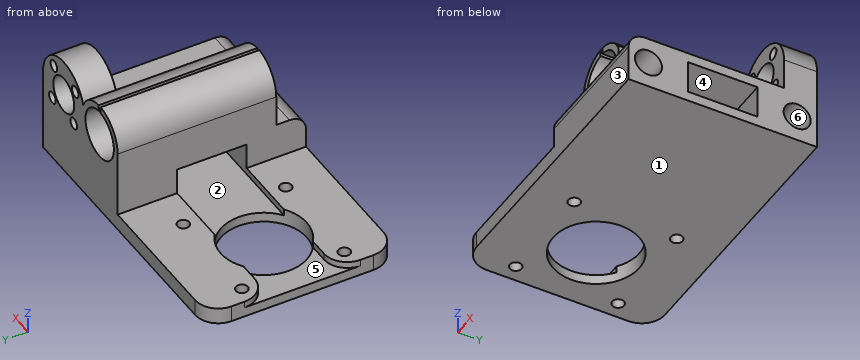
from build123d import *

# Parameters (mm, degrees)
SKETCH2_R             = 5.5
SKETCH2_R_2           = 1.75
BOSS_EXTRUDE1_DEPTH   = 28.5
CUT_EXTRUDE1_START    = 16
CUT_EXTRUDE1_DEPTH    = 83.998737366
SKETCH4_R             = 1.8
SKETCH4_R_2           = 13
HOLES_FOR_MOTOR_DEPTH = 99.998737366
SKETCH6_W             = 10
SKETCH6_H             = 21
CUT_EXTRUDE3_DEPTH    = 99.998737366
SKETCH11_R            = 4.1
CUT_EXTRUDE7_DEPTH    = 21.691
FILLET2_R             = 5
FILLET3_R             = 7


with BuildPart() as part:
    # Sketch2 → Boss-Extrude1 (new, symmetric)
    with BuildSketch(Plane(origin=(0, 0, 0), x_dir=(1, 0, 0), z_dir=(0, 1, 0))):
        with BuildLine():
            Line((58, -34.986832981), (58, -32.983314774))
            ThreePointArc((58, -32.983314774), (57.5, -18), (57, -32.983314774))
            Line((57, -32.983314774), (57, -34.986832981))
            ThreePointArc((57, -34.986832981), (50.607975624, -32.038348415), (48, -25.5))
            Line((48, -25.5), (48, -5))
            Line((48, -5), (0, -5))
            Line((0, -5), (0, 0))
            Line((0, 0), (87.5, 0))
            Line((87.5, 0), (87.5, -25.5))
            ThreePointArc((87.5, -25.5), (78.449190115, -36.325925267), (66.190789474, -29.336688458))
            ThreePointArc((66.190789474, -29.336688458), (62.894319797, -33.319930558), (58, -34.986832981))
        make_face()
        with Locations(Location((76.5, -25.5, 0), (0, 0, 90))):
            Circle(SKETCH2_R, mode=Mode.SUBTRACT)
        with Locations(Location((70.462323358, -30.748472232, 0), (0, 0, 90))):
            Circle(SKETCH2_R_2, mode=Mode.SUBTRACT)
        with Locations(Location((82.537676642, -20.251527768, 0), (0, 0, 90))):
            Circle(SKETCH2_R_2, mode=Mode.SUBTRACT)
        with Locations(Location((71.251527768, -19.462323358, 0), (0, 0, 90))):
            Circle(SKETCH2_R_2, mode=Mode.SUBTRACT)
        with Locations(Location((81.748472232, -31.537676642, 0), (0, 0, 90))):
            Circle(SKETCH2_R_2, mode=Mode.SUBTRACT)
    extrude(amount=BOSS_EXTRUDE1_DEPTH, both=True)

    # Sketch3 → Cut-Extrude1 (cut, through all)
    with BuildSketch(Plane.XY.offset(CUT_EXTRUDE1_START)):
        Polygon((66.4, 18.5), (88, 18.5), (88, -28.5), (48, -28.5), (48, -19.5), (66.4, -19.5), align=None)
    extrude(amount=CUT_EXTRUDE1_DEPTH, mode=Mode.SUBTRACT)

    # Sketch4 → Holes-for-motor (cut, through all)
    with BuildSketch(Plane.XY):
        with Locations(Location((5, 15.5, 0), (0, 0, 180))):
            Circle(SKETCH4_R)
        with Locations(Location((36, 15.5, 0), (0, 0, 180))):
            Circle(SKETCH4_R)
        with Locations(Location((5, -15.5, 0), (0, 0, 180))):
            Circle(SKETCH4_R)
        with Locations(Location((36, -15.5, 0), (0, 0, 180))):
            Circle(SKETCH4_R)
        with Locations(Location((20.5, 0, 0), (0, 0, 180))):
            Circle(SKETCH4_R_2)
    extrude(amount=HOLES_FOR_MOTOR_DEPTH, mode=Mode.SUBTRACT)

    # Sketch6 → Cut-Extrude3 (cut, through all)
    with BuildSketch(Plane(origin=(0, 0, 0), x_dir=(0, 0, -1), z_dir=(1, 0, 0))):
        with Locations((-8, 0)):
            Rectangle(SKETCH6_W, SKETCH6_H)
    extrude(amount=CUT_EXTRUDE3_DEPTH, mode=Mode.SUBTRACT)

    # Sketch11 → Cut-Extrude7 (cut)
    with BuildSketch(Plane(origin=(87.5, 0, 0), x_dir=(0, 0, -1), z_dir=(1, 0, 0))):
        with Locations((-8, -22.5)):
            Circle(SKETCH11_R)
        with Locations((-8, 22.5)):
            Circle(SKETCH11_R)
    extrude(amount=-CUT_EXTRUDE7_DEPTH, mode=Mode.SUBTRACT)

    # Fillet2
    fillet2_edges = [part.edges().sort_by_distance(p)[0] for p in [
        (67.75, -28.5, 16),
    ]]
    fillet(fillet2_edges, radius=FILLET2_R)

    # Fillet3
    fillet3_edges = [part.edges().sort_by_distance(p)[0] for p in [
        (0, -10.5, 4),
        (0, 10.5, 4),
        (0, -28.5, 2.5),
        (0, 28.5, 2.5),
    ]]
    fillet(fillet3_edges, radius=FILLET3_R)


solid = part.part
Design review of the part built by this model. Coordinates are the model's own, in mm. Face numbers are marked on the shaded views. A direction names the side the tool comes from. Give positions to 0.01 mm unless a question says otherwise; leave off trailing zeros. Loops run counter-clockwise (first coordinate to the right, second up) from the corner with the lowest first, then second, coordinate; pieces in that order, holes last. Notation, with made-up numbers: M 26.5,-15 L 77.5,-15 A4 ccw 77.5,-9 Z; hole C -22.75,44 d2. An arc over 180 degrees is marked long. Answer as a JSON object with one key per item and string values.
Item 1: Wall thickness on line 1 along Y through (x, z) = (51, 10); line 2 along Z through (x, y) = (72, 8.5); line 3 along X through (y, z) = (15.5, 2.4): over which ranges is each line inside the solid? List them lowest first.
Output values:
{"line 1": "y = -28.5 to -10.5, 10.5 to 28.5", "line 2": "z = 0 to 3, 13 to 16", "line 3": "x = 0 to 3.2, 6.8 to 34.2, 37.8 to 87.5"}
Item 2: We need section C-C (x = 52). State the section outline as (y, z) points, and give its area (3 significant figures).
Output values:
{"outline": "M -28.5,0 L 28.5,0 L 28.5,20.4 L -19.5,20.4 L -19.5,16 L -23.5,16 A5 ccw -28.5,11 Z; M -19.5,30.6 L 28.5,30.6 L 28.5,33.25 L -19.5,33.25 Z; hole M -10.5,3 L 10.5,3 L 10.5,13 L -10.5,13 Z", "area": "1,030 mm2"}
Item 3: For P1, Ø2, axis at x = 36, y = -15.5, coming from the +Z side; P2, Ø9, axis at x = 15, y = -19.5, coming from the +Z side; P3, Ø0.6, axis at y = 16, z = 34.5, coming from the +X side; P4, Ø12, axis at x = 77.5, z = 18, coming from the -Y side, all flat-tipped, find the tip position at first contact; note any pin that passes through.
Output values:
{"P1": "passes through", "P2": "stops at z = 5", "P3": "stops at x = 61.32", "P4": "stops at y = -28.4"}
Item 4: We need section D-D (y = 3.5). State the section outline as (x, z) points.
Output values:
{"outline": "M 0,0 L 7.98,0 L 7.98,3 L 0,3 Z; M 33.02,0 L 87.5,0 L 87.5,3 L 33.02,3 Z; M 48,13 L 87.5,13 L 87.5,16 L 66.4,16 L 66.4,29.86 A11 ccw 66.19,29.34 A9.5 ccw 58,34.99 L 58,32.98 A7.5 cw long 57,32.98 L 57,34.99 A9.5 ccw 48,25.5 Z"}
Item 5: Mouldability with a two-part tool opening along Y and no side actions: class the marked faces 1, 2 and 3 as pulls with the +Y half, pulls with the -Y half, needs draft (parallel to the pull), parting line crosses it, or undercut.
Output values:
{"face 1": "needs draft", "face 2": "undercut", "face 3": "pulls with the -Y half"}
Item 6: Machinability: for the marked faces 4, 5 and 6, which of the approach directions +Z, -Z, +X, -X, +Y, -Y give a long, thin tool a straight path to every point of the face, cutting with its end or side? Answer none if there is none.
Output values:
{"face 4": "+X, -X", "face 5": "+Z, -X", "face 6": "+X"}
Item 7: We need section B-B (z = 8). State the section outline as (x, y) points.
Output values:
{"outline": "M 48,-28.5 L 87.5,-28.5 L 87.5,-26.6 L 65.81,-26.6 L 65.81,-18.4 L 87.5,-18.4 L 87.5,-10.5 L 48,-10.5 Z; M 48,10.5 L 87.5,10.5 L 87.5,18.4 L 65.81,18.4 L 65.81,26.6 L 87.5,26.6 L 87.5,28.5 L 48,28.5 Z"}
Item 8: We need section A-A (x = 76.5). State the section outline as (y, z) points.
Output values:
{"outline": "M -28.5,0 L 28.5,0 L 28.5,20 L 18.5,20 L 18.5,16 L -23.5,16 A5 ccw -28.5,11 Z; M 18.5,31 L 28.5,31 L 28.5,36.5 L 18.5,36.5 Z; hole C -22.5,8 d8.2; hole M -10.5,3 L 10.5,3 L 10.5,13 L -10.5,13 Z; hole C 22.5,8 d8.2"}
